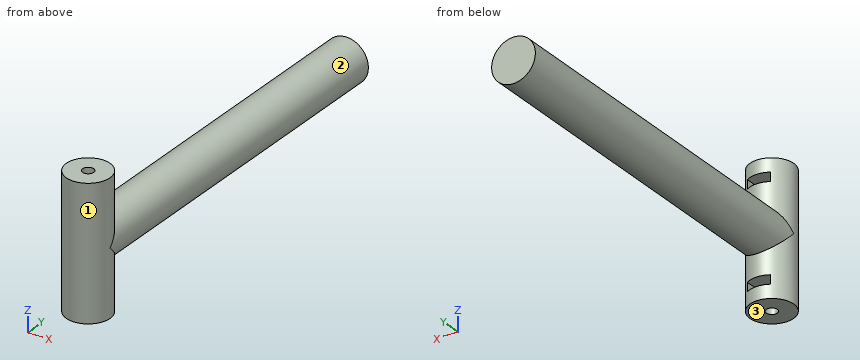
```python
from build123d import *

# Parameters (mm, degrees)
BOSS_EXTRUDE1_DEPTH      = 14.8
BOSS_EXTRUDE1_DEPTH_BACK = 14.8
SKETCH1_R                = 4.9
SKETCH2_R                = 4.9
BOSS_EXTRUDE2_DEPTH      = 84
CUT_EXTRUDE1_DEPTH       = 2
SKETCH5_W                = 5.196152422
SKETCH5_H                = 2
CUT_EXTRUDE2_DEPTH       = 12
SKETCH6_R                = 1.25
CUT_EXTRUDE3_DEPTH       = 10


with BuildPart() as part:
    # Sketch1 → Boss-Extrude1 (new, two sides: drawn at the far end of the back side and taken through both)
    with BuildSketch(Plane.XY.offset(-BOSS_EXTRUDE1_DEPTH_BACK)):
        Circle(SKETCH1_R)
    extrude(amount=BOSS_EXTRUDE1_DEPTH + BOSS_EXTRUDE1_DEPTH_BACK)

    # Sketch2 → Boss-Extrude2 (add)
    with BuildSketch(Plane(origin=(0, 0, 0), x_dir=(1, 0, 0), z_dir=(0, 1, 0))):
        Circle(SKETCH2_R)
    extrude(amount=BOSS_EXTRUDE2_DEPTH)

    # Sketch4 → Cut-Extrude1 (cut)
    with BuildSketch(Plane.XY.offset(11.8)):
        Polygon((2.598076211, 0), (1.299038106, 2.25), (-1.299038106, 2.25), (-2.598076211, 0), (-1.299038106, -2.25), (1.299038106, -2.25), align=None)
    cut_extrude1 = extrude(amount=-CUT_EXTRUDE1_DEPTH, mode=Mode.SUBTRACT)

    # Sketch5 → Cut-Extrude2 (cut)
    with BuildSketch(Plane(origin=(0, 0, 0), x_dir=(1, 0, 0), z_dir=(0, 1, 0))):
        with Locations((0, -10.8)):
            Rectangle(SKETCH5_W, SKETCH5_H)
    cut_extrude2 = extrude(amount=CUT_EXTRUDE2_DEPTH, mode=Mode.SUBTRACT)

    # Mirror2: Cut-Extrude1, Cut-Extrude2 across plane
    add(cut_extrude1.mirror(Plane.XY), mode=Mode.SUBTRACT)
    add(cut_extrude2.mirror(Plane.XY), mode=Mode.SUBTRACT)

    # Sketch6 → Cut-Extrude3 (cut)
    with BuildSketch(Plane(origin=(0, 0, -14.8), x_dir=(-1, 0, 0), z_dir=(0, 0, -1))):
        Circle(SKETCH6_R)
    cut_extrude3 = extrude(amount=-CUT_EXTRUDE3_DEPTH, mode=Mode.SUBTRACT)

    # Mirror3: Cut-Extrude3 across plane
    add(cut_extrude3.mirror(Plane.XY), mode=Mode.SUBTRACT)


solid = part.part
```
Check sheet for the modelled part. Datum: model origin and axes. Units: mm. Face numbers are marked on the shaded views. A direction names the side the tool comes from. Round coordinates to 2 decimals unless told otherwise and drop trailing zeros. Order: outer loops, then holes, each group sorted by start corner. A loop starts at its lowest first (then second) coordinate and runs counter-clockwise, first axis right, second up. Notation, with made-up numbers: (53.5, 25) - (104.5, 25) arc R30 cw to (104.5, 52) - close; hole circle Ø7 at (73.5, -21). An arc over 180 degrees is marked (long way). Write item = value, one per line.
Q1. Thickness scan on line 1 along Y through (x, z) = (0, 13.25); line 2 along Z through (x, y) = (-1, 42). Record the ranges inside material, lowest first.
Computed:
line_1 = -4.9 to -1.25, 1.25 to 4.9
line_2 = -4.8 to 4.8
Q2. Section check C-C (y = 72.5). Record the boundary of the cut face in (x, z).
Computed:
outline = circle Ø9.8 at (0, 0)
Q3. Section check A-A (x = 0). State how many separate pieces and enclosed holes the cut face has, and give its area (3 significant figures).
Computed:
separate_pieces = 3
enclosed_holes = 0
area = 997 mm^2
Q4. Section check B-B (x = 3.5). Record the boundary of the cut face in (y, z).
Computed:
outline = (-3.43, -14.8) - (3.43, -14.8) - (3.43, -3.43) - (84, -3.43) - (84, 3.43) - (3.43, 3.43) - (3.43, 14.8) - (-3.43, 14.8) - close
Q5. Tool access check on the marked faces 1, 2 and 3. Record the directions out of +Z, -Z, +X, -X, +Y, -Y that give a thin tool (end or side, any length) a straight path to the whole face; none if there is none.
Computed:
face_1 = none
face_2 = +Y
face_3 = -Z, +X, -X, +Y, -Y
Q6. Section check D-D (z = -1). Record the boundary of the cut face in (x, y).
Computed:
outline = (-4.8, 1) arc R4.9 ccw (long way) to (4.8, 1) - (4.8, 84) - (-4.8, 84) - close
Q7. Go/stop test with flat-tipped pins: pin 1 (1 mm diameter, centred on y = 3, z = -11, fed in from -X); pin 2 (3 mm diameter, centred on x = 1.5, z = 3, fed in from -Y); pin 3 (1.6 mm diameter, centred on y = 2.5, z = -11, fed in from +X); pin 4 (1.5 mm diameter, centred on x = 0, y = 0, fed in from +Z). Record where each tip stops, or that it passes through.
Computed:
pin_1 = -4.21
pin_2 = -4.9
pin_3 = 4.6
pin_4 = 4.8
